Check sheet for the drawn part. Datum: minimum x, y, z corner. Units: mm. Give positions to 0.01 mm unless a question says otherwise; leave off trailing zeros. Loops run counter-clockwise (first coordinate to the right, second up) from the corner with the lowest first, then second, coordinate; pieces in that order, holes last. Notation, with made-up numbers: (34.5, -12) - (61.5, -12) arc R20 ccw to (61.5, 5) - close; hole circle Ø9 at (22.5, 71.5). An arc over 180 degrees is marked (long way). Use one line per item in the form item = value.
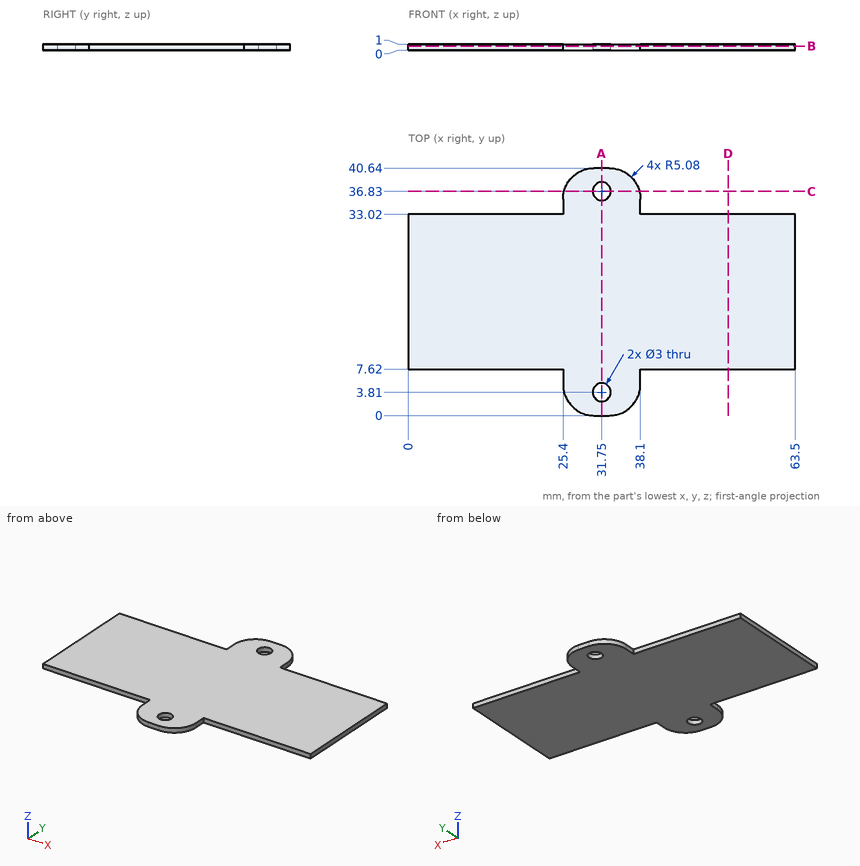
1. Section check A-A, the plane x = 31.75. Record the cut outline in (y, z).
Result set:
outline = (0, 0) - (2.31, 0) - (2.31, 1) - (0, 1) - close; (5.31, 0) - (35.33, 0) - (35.33, 1) - (5.31, 1) - close; (38.33, 0) - (40.64, 0) - (40.64, 1) - (38.33, 1) - close
2. Section check B-B, the plane z = 0.65. Record the cut outline in (x, y).
Result set:
outline = (0, 7.62) - (25.4, 7.62) - (25.4, 5.08) arc R5.08 ccw to (30.48, 0) - (33.02, 0) arc R5.08 ccw to (38.1, 5.08) - (38.1, 7.62) - (63.5, 7.62) - (63.5, 33.02) - (38.1, 33.02) - (38.1, 35.56) arc R5.08 ccw to (33.02, 40.64) - (30.48, 40.64) arc R5.08 ccw to (25.4, 35.56) - (25.4, 33.02) - (0, 33.02) - close; hole circle Ø3 at (31.75, 3.81); hole circle Ø3 at (31.75, 36.83)
3. Depth check by flat-ended pin: pin 1 Ø0.5 at (x, z) = (8.5, 0.5) entering from +Y; pin 2 Ø0.5 at (y, z) = (35, 0.5) entering from -X; pin 3 Ø0.5 at (y, z) = (33.5, 0.5) entering from +X. Enter the tip coordinate at first touch or a pass-through.
Result set:
pin_1 = 33.02
pin_2 = 25.4
pin_3 = 38.1
4. Section check C-C, the plane y = 36.83. Record the cut outline in (x, z).
Result set:
outline = (25.56, 0) - (30.25, 0) - (30.25, 1) - (25.56, 1) - close; (33.25, 0) - (37.94, 0) - (37.94, 1) - (33.25, 1) - close
5. Section check D-D, the plane x = 52.5. Record the cut outline in (y, z), then the cut area to 3 significant figures.
Result set:
outline = (7.62, 0) - (33.02, 0) - (33.02, 1) - (7.62, 1) - close
area = 25.4 mm²
6. Scan lines: probe 1 along Y at (x, z) = (18, 0.1); probe 2 along X at (y, z) = (37, 0.8); probe 3 along X at (y, z) = (35.5, 0.6). Record each from-to range of solid material in increasing order.
Result set:
probe_1 = 7.62 to 33.02
probe_2 = 25.61 to 30.26, 33.24 to 37.89
probe_3 = 25.4 to 31.06, 32.44 to 38.1
